```python
from build123d import *

# Parameters (mm, degrees)
SKETCH1_R           = 15
BOSS_EXTRUDE1_DEPTH = 14.75
CUT_EXTRUDE1_DEPTH  = 15.75
CIRPATTERN1_COUNT   = 10


with BuildPart() as part:
    # Sketch1 → Boss-Extrude1 (new body)
    with BuildSketch(Plane.XY):
        Circle(SKETCH1_R)
    extrude(amount=BOSS_EXTRUDE1_DEPTH)

    # Sketch2 → Cut-Extrude1 (cut, through all)
    with BuildSketch(Plane.XY.offset(14.75)):
        with BuildLine():
            ThreePointArc((-1.25, 8.912771735), (0, 9), (1.25, 8.912771735))
            ThreePointArc((1.25, 8.912771735), (2.05890341, 12.07109765), (4.4, 14.340153416))
            ThreePointArc((4.4, 14.340153416), (0, 15), (-4.4, 14.340153416))
            ThreePointArc((-4.4, 14.340153416), (-2.05890341, 12.07109765), (-1.25, 8.912771735))
        make_face()
    cut_extrude1 = extrude(amount=-CUT_EXTRUDE1_DEPTH, mode=Mode.SUBTRACT)

    # CirPattern1: Cut-Extrude1 ×10 about axis
    cirpattern1_axis = Axis((0, 0, 0), (0, 0, 1))
    for i in range(1, CIRPATTERN1_COUNT):
        add(cut_extrude1.rotate(cirpattern1_axis, i * 360 / CIRPATTERN1_COUNT), mode=Mode.SUBTRACT)


solid = part.part
```
Could you check a few things on this model? Use its own coordinates, in mm. A direction names the side the tool comes from. Give positions to 0.01 mm unless a question says otherwise; leave off trailing zeros. Write each loop counter-clockwise with the first axis right and the second up, starting at its lowest first coordinate (ties: lowest second). Pieces come first, ordered by that corner, then holes. Notation, with made-up numbers: (1.5, -32.5) - (54.5, -32.5) arc R20 ccw to (54.5, -26.5) - close; hole circle Ø8 at (33.25, 26.25). An arc over 180 degrees is marked (long way). One line per item, written item: value. Start each with the question number.
Item 1: Imagine slicing it at A-A, the plane y = 7. List the corners of the cut face in (x, z) for me, and give its area (3 significant figures).
Item 2: Please list where these lines run through material, in increasing order: line 1 (Y direction, x = 11, z = 5.75); line 2 (X direction, y = -7.25, z = 4.5); line 3 (X direction, y = -8.5, z = 5.75). Write a range as from..to.
Item 3: Imagine slicing it at B-B, the plane y = 10.5. List the corners of the cut face in (x, z) for me.
Item 4: Imagine slicing it at D-D, the plane y = -12.5. List the corners of the cut face in (x, z) for me.
Item 5: Imagine slicing it at C-C, the plane x = -11. List the corners of the cut face in (y, z) for me, and give its area (3 significant figures).
Item 6: Which directions (+Z, -Z, +X, -X, +Y, -Y) give clear straight access to the entire face, cutting with the end or side of a thin tool? Please do faces 3 (the face through (0, 0, 0)), 4 (the face through (12.07, 1.78, 7.48)).
Item 7: I'm going to push flat-ended pins straight in: pin 1 (8 mm diameter, centred on y = -5, z = 9, fed in from -X); pin 2 (8 mm diameter, centred on x = -6.5, y = -9, fed in from -Z); pin 3 (3 mm diameter, centred on y = -8.5, z = 12.5, fed in from -X); pin 4 (2 mm diameter, centred on x = 11, z = 4, fed in from -Y). Where does each tip first touch, or does it pass through?
Item 8: If we mould it in two halves opening along X, with no side actions, what happens to faces 1 (the face through (2.036, 12.031, 7.478)), 2 (the face through (0, 0, 14.75))? For each: +X half, -X half, draft (parallel to the pull), parting line (faces both ways), or undercut.
Geometry says:
1. outline: (-11.74, 0) - (-6.66, 0) - (-6.66, 14.75) - (-11.74, 14.75) - close; (-5.66, 0) - (5.66, 0) - (5.66, 14.75) - (-5.66, 14.75) - close; (6.66, 0) - (11.74, 0) - (11.74, 14.75) - (6.66, 14.75) - close
1. area: 317 mm^2
2. line 1: -9.07..-5.87, -1.9..1.9, 5.87..9.07
2. line 2: -11.86..-6.89, -5.33..5.33, 6.89..11.86
2. line 3: -12.26..-8.64, -4.6..4.6, 8.64..12.26
3. outline: (-5.36, 0) - (-1.42, 0) - (-1.42, 14.75) - (-5.36, 14.75) - close; (1.42, 0) - (5.36, 0) - (5.36, 14.75) - (1.42, 14.75) - close
4. outline: (-5.39, 0) - (-2.33, 0) - (-2.33, 14.75) - (-5.39, 14.75) - close; (2.33, 0) - (5.39, 0) - (5.39, 14.75) - (2.33, 14.75) - close
5. outline: (-9.07, 0) - (-5.87, 0) - (-5.87, 14.75) - (-9.07, 14.75) - close; (-1.9, 0) - (1.9, 0) - (1.9, 14.75) - (-1.9, 14.75) - close; (5.87, 0) - (9.07, 0) - (9.07, 14.75) - (5.87, 14.75) - close
5. area: 150 mm^2
6. face 3: -Z, +X, -X, +Y, -Y
6. face 4: +Z, -Z
7. pin 1: x = -14.03
7. pin 2: z = 0
7. pin 3: x = -12.28
7. pin 4: y = -9.07
8. face 1: undercut
8. face 2: draft
